Autodesk Inventor part; units mm, degrees
ref_plane "YZ Plane" through (0, 0, 0) normal (1, 0, 0) x (0, 1, 0)
ref_plane "XZ Plane" through (0, 0, 0) normal (0, 1, 0) x (-1, 0, 0)
ref_plane "XY Plane" through (0, 0, 0) normal (0, 0, 1) x (1, 0, 0)
sketch "Sketch1" plane through (0, 0, 0) normal (0, 0, 1) x (1, 0, 0)
  line L0 (-6.0954, 5.4228) -> (18.9046, 5.4228)
  line L1 (18.9046, 5.4228) -> (18.9046, -19.5772)
  line L2 (18.9046, -19.5772) -> (-6.0954, -19.5772)
  line L3 (-6.0954, -19.5772) -> (-6.0954, 5.4228)
  line L4 (-6.0954, -22.5772) -> (21.9046, -22.5772)
  line L5 (21.9046, -22.5772) -> (21.9046, 5.4228)
  line L6 (18.9046, 5.4228) -> (21.9046, 5.4228)
  line L7 (-6.0954, -19.5772) -> (-6.0954, -22.5772)
  line L8 (18.9046, -19.5772) -> (18.9046, -22.5772)
  point P0 (0, 0)
  point P1 (6.4046, -7.0772)
  dimension "d0" = 25
  dimension "d1" = 25
  dimension "d2" = 3
  dimension "d3" = 3
  dimension "d4" = 12.5
  dimension "d5" = 12.5
extrude "Extrusion1" add sketch "Sketch1" along normal blind 6
extrude "Extrusion2" add sketch "Sketch1" against normal blind 2 contours L6 L5 L4 L8 L1 | L2 L8 L4 L7
hole "Hole1" at (6.4046, -7.0772, 0) direction (0, 0, 1) diameter 4 end through all
sketch "Sketch2" plane through (0, 0, 6) normal (0, 0, 1) x (1, 0, 0)
  circle A0 centre (6.4046, -7.0772) radius 2
  line L0 (-6.0954, 5.4228) -> (-6.0954, -22.5772)
  line L1 (-6.0954, -22.5772) -> (21.9046, -22.5772)
  line L2 (21.9046, -22.5772) -> (21.9046, 5.4228)
  line L3 (21.9046, 5.4228) -> (-6.0954, 5.4228)
  circle A1 centre (6.4046, -7.0772) radius 2
  circle A2 centre (6.4046, -7.0772) radius 4.5
  point P0 (0, 0)
  dimension "d17" = 9
extrude "Extrusion3" cut sketch "Sketch2" against normal blind 1.5 contours A2
chamfer "Chamfer1" distance 2 angle 45 1 edges at (6.4046, -9.0772, 4.5)
sketch "Sketch3" plane through (0, 0, -2) normal (0, 0, -1) x (-1, 0, 0)
  line L0 (6.0954, -19.5772) -> (-18.9046, -19.5772)
  line L1 (-18.9046, -19.5772) -> (-18.9046, 5.4228)
  line L2 (-18.9046, 5.4228) -> (-21.9046, 5.4228)
  line L3 (-21.9046, 5.4228) -> (-21.9046, -22.5772)
  line L4 (-21.9046, -22.5772) -> (6.0954, -22.5772)
  line L5 (6.0954, -22.5772) -> (6.0954, -19.5772)
  line L6 (-18.9046, 5.4228) -> (-21.9046, 5.4228)
  line L7 (-21.9046, 5.4228) -> (-18.9046, 5.4228)
  line L8 (-18.9046, 5.4228) -> (-18.9046, -22.5772)
  line L9 (-18.9046, -22.5772) -> (-21.9046, -22.5772)
  line L10 (-21.9046, -22.5772) -> (-21.9046, 5.4228)
  point P0 (0, 0)
extrude "Extrusion4" cut sketch "Sketch3" against normal through all contours L8 L4 L3 L2 L1
fillet "Fillet2" radius 2 3 edges at (18.9046, -22.5772, 2) (-6.0954, 5.4228, 3) (18.9046, 5.4228, 3)
properties part number "3DP_PLA_Base_plate_side_leg" material "ABS Plastic"
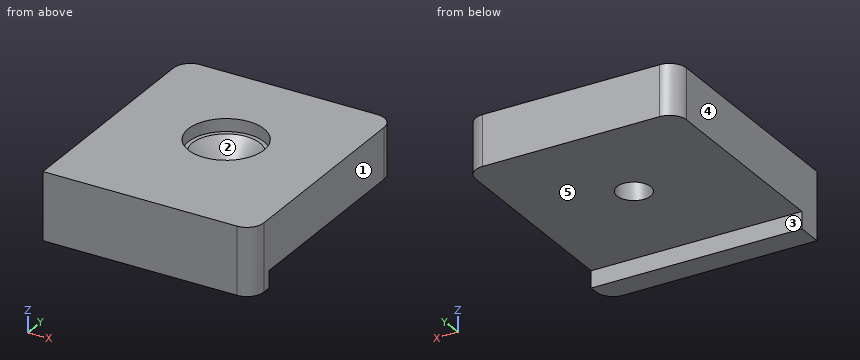
Input: part model. Units: mm. Frame: model coordinates. Face numbers are marked on the shaded views. A direction names the side the tool comes from. Round coordinates to 2 decimals unless told otherwise and drop trailing zeros. Order: outer loops, then holes, each group sorted by start corner. A loop starts at its lowest first (then second) coordinate and runs counter-clockwise, first axis right, second up. Notation, with made-up numbers: (17, -20.75) - (29, -20.75) arc R21 ccw to (29, -6.75) - close; hole circle Ø5 at (38, -23). An arc over 180 degrees is marked (long way). Answer in a Markdown table with one row per item.
Item 1: Section query B-B (z = -0.75). Return the cut outline in (x, y).
Model answer:
| item | result |
|---|---|
| outline | (-6.1, -22.58) - (16.9, -22.58) arc R2 ccw to (18.9, -20.58) - (18.9, -19.58) - (-6.1, -19.58) - close |
Item 2: Section query C-C (x = -3). Return the cut outline in (y, z).
Model answer:
| item | result |
|---|---|
| outline | (-22.58, -2) - (-19.58, -2) - (-19.58, 0) - (5.42, 0) - (5.42, 6) - (-22.58, 6) - close |
Item 3: Line query: line 1 (Y direction, x = 6.5, z = 0.5); line 2 (Z direction, x = -1.25, y = 2.5); line 3 (Y direction, x = 0, z = -0.25). Output: solid intervals per line, ascending.
Model answer:
| item | result |
|---|---|
| line 1 | y = -22.58 to -9.07, -5.08 to 5.42 |
| line 2 | z = 0 to 6 |
| line 3 | y = -22.58 to -19.58 |
Item 4: Reachability of the marked faces 4 and 5 from +Z, -Z, +X, -X, +Y, -Y: full face, straight path, thin tool, end or side. Return the list, or none.
Model answer:
| item | result |
|---|---|
| face 4 | +Z, -Z, -X, +Y, -Y |
| face 5 | -Z, +X, -X, +Y |
Item 5: Section query D-D (y = -17). Return the cut outline in (x, z), then the cut area to 3 significant figures.
Model answer:
| item | result |
|---|---|
| outline | (-6.1, 0) - (18.9, 0) - (18.9, 6) - (-6.1, 6) - close |
| area | 150 mm² |
Item 6: Section query A-A (z = 4). Return the cut outline in (x, y), then the cut area to 3 significant figures.
Model answer:
| item | result |
|---|---|
| outline | (-6.1, -22.58) - (16.9, -22.58) arc R2 ccw to (18.9, -20.58) - (18.9, 3.42) arc R2 ccw to (16.9, 5.42) - (-4.1, 5.42) arc R2 ccw to (-6.1, 3.42) - close; hole circle Ø7 at (6.4, -7.08) |
| area | 659 mm² |
Item 7: Mould query, pull axis X, two halves, no side actions, for the marked faces 1, 2 and 3. Classes: released by +X, released by -X, zero draft, split by the parting line, or undercut.
Model answer:
| item | result |
|---|---|
| face 1 | released by +X |
| face 2 | undercut |
| face 3 | zero draft |
Item 8: Pin query (flat end, axial travel): pin 1 (4 mm diameter, centred on x = 5, y = -6.5, fed in from -Z); pin 2 (1 mm diameter, centred on x = 0.5, z = -1, fed in from +Y); pin 3 (4.5 mm diameter, centred on x = 6.5, y = -5, fed in from +Z). Return the tip coordinate at first contact, or that it passes through.
Model answer:
| item | result |
|---|---|
| pin 1 | stops at z = 0 |
| pin 2 | stops at y = -19.58 |
| pin 3 | stops at z = 4.5 |
